from build123d import *

# Parameters (mm, degrees)
BOSS_EXTRUDE1_DEPTH = 3.15
SKETCH2_R           = 2.45
BOSS_EXTRUDE2_DEPTH = 1.8
SHELL1_T            = -1.5


with BuildPart() as part:
    # Sketch1 → Boss-Extrude1 (new body)
    with BuildSketch(Plane.XY):
        Polygon((0, 0), (23.85, 0), (23.85, 8.09), (0, 15.85), align=None)
    extrude(amount=-BOSS_EXTRUDE1_DEPTH)

    # Sketch2 → Boss-Extrude2 (add)
    with BuildSketch(Plane.XY):
        with Locations((3.975, 4.045)):
            Circle(SKETCH2_R)
        with Locations((11.925, 4.045)):
            Circle(SKETCH2_R)
        with Locations((19.875, 4.045)):
            Circle(SKETCH2_R)
    extrude(amount=BOSS_EXTRUDE2_DEPTH)

    # Shell1
    shell1_openings = [part.faces().sort_by_distance(p)[0] for p in [
        (10.636528822, 6.194612921, -3.15),
    ]]
    offset(amount=SHELL1_T, openings=shell1_openings, kind=Kind.INTERSECTION)


solid = part.part
Design review of the part built by this model. Coordinates are the model's own, in mm. A direction names the side the tool comes from. Give positions to 0.01 mm unless a question says otherwise; leave off trailing zeros. Loops run counter-clockwise (first coordinate to the right, second up) from the corner with the lowest first, then second, coordinate; pieces in that order, holes last. Notation, with made-up numbers: M 70.25,-36 L 79.25,-36 A31 ccw 79.25,3 Z; hole C 15.5,14 d11. An arc over 180 degrees is marked long. Write item = value, one per line.
Q1. We need section C-C (y = 8.75). Give the boundary of the cut face in (x, z), plus the area to 3 significant figures.
Output values:
outline = M 0,-3.15 L 1.5,-3.15 L 1.5,-1.5 L 16.97,-1.5 L 16.97,-3.15 L 21.82,-3.15 L 21.82,0 L 0,0 Z
area = 43.2 mm^2
Q2. We need section D-D (x = 16). Give the boundary of the cut face in (y, z), plus the area to 3 significant figures.
Output values:
outline = M 0,-3.15 L 1.5,-3.15 L 1.5,-1.5 L 9.07,-1.5 L 9.07,-3.15 L 10.64,-3.15 L 10.64,0 L 0,0 Z
area = 21.0 mm^2
Q3. Draft analysis for pull direction Y (two halves, no side actions). For faces 4 (the cylindrical face through (14.19, 3.11, 0.89)), 5 (the flat face through (12, 4, 0.3)), 6 (the flat face through (12.092, 11.916, -1.553)), 7 (the flat face through (20, 4, 1.8)), state which applies: +Y half, -Y half, draft (parallel to the pull), parting line (faces both ways), or undercut.
Output values:
face_4 = parting line
face_5 = undercut
face_6 = +Y half
face_7 = draft
Q4. Insertion check: pin 1 (1.5 mm diameter, centred on x = 20, y = 4.5, fed in from -Z); pin 2 (2 mm diameter, centred on x = 6, z = 0, fed in from +Y); pin 3 (1.5 mm diameter, centred on x = 12, y = 4, fed in from -Z). Each pin has a flat end and moves straight along its axis. Give the tip position at first contact, or say it passes through.
Output values:
pin_1 = -1.5
pin_2 = 14.22
pin_3 = 0.3
Q5. For faces 1 (the flat face through (22.35, 4, -2)), 2 (the flat face through (0, 8, -2)), 3 (the cylindrical face through (17.931, 2.554, 0.887)), list the 3-axis set-ups (+Z, -Z, +X, -X, +Y, -Y) from which the entire face can be reached by the end or side of a thin tool; tool diameter is ignored.
Output values:
face_1 = -Z
face_2 = +Z, -Z, -X, +Y, -Y
face_3 = +Z
Q6. We need section B-B (z = -0.6). Give the boundary of the cut face in (x, y) (3 decimals).
Output values:
outline = M 0,0 L 23.85,0 L 23.85,8.09 L 0,15.85 Z; hole C 3.975,4.045 d1.9; hole C 11.925,4.045 d1.9; hole C 19.875,4.045 d1.9
Q7. To check wall thickness, follow line 1 (X direction, y = 4.75, z = -1.65); line 2 (X direction, y = 2, z = 0.65); line 3 (Z direction, x = 2.75, y = 1). State the ranges of each line that lie inside material, in increasing order. Write a range as [from, to].
Output values:
line_1 = [0, 1.5], [22.35, 23.85]
line_2 = [2.63, 5.32], [10.58, 13.27], [18.53, 21.22]
line_3 = [-3.15, 0]
Q8. We need section A-A (z = -2.05). Give the boundary of the cut face in (x, y), plus the area to 3 significant figures.
Output values:
outline = M 0,0 L 23.85,0 L 23.85,8.09 L 0,15.85 Z; hole M 1.5,1.5 L 22.35,1.5 L 22.35,7 L 1.5,13.78 Z
area = 100 mm^2
